Read the model definition and answer for the solid it produces. Units are mm, in the model's axes. Face numbers are marked on the shaded views. A direction names the side the tool comes from. Coordinates: 2 decimals unless noted, no trailing zeros. Write each loop counter-clockwise with the first axis right and the second up, starting at its lowest first coordinate (ties: lowest second). Pieces come first, ordered by that corner, then holes.
Item 1: Section C-C (z = -3.5) is taken. Give the vertices of the cut face in (x, y).
Item 2: Straight lines are drawn through the part: probe 1 along Y at (x, z) = (3.5, 2); probe 2 along X at (y, z) = (-30, 7.75); probe 3 along X at (y, z) = (24, 6). For each, find the intervals that lie inside material, in ascending order.
Item 3: Section D-D (x = -20) is taken. Give the vertices of the cut face in (y, z), then the cut area to 3 significant figures.
Item 4: Section A-A (z = 8.5) is taken. State how many separate pieces and enclosed holes the cut face has, then the cut area to 3 significant figures.
Item 5: Determine the mould class of the marked faces 6, 7, 8 and 9 for opening direction X: released by +X, released by -X, zero draft, split by the parting line, or undercut.
Item 6: A tool of negligible diameter and unlimited length cuts with its end or side. For the marked faces 1, 2, 3, 4 and 5, from which of +Z, -Z, +X, -X, +Y, -Y can it reach the whole face along a straight path? Write none if from no direction.
Item 7: Each of these flat-tipped pins is pushed along its axis until it touches: P1, Ø6, axis at x = -20, y = -30, coming from the +Z side; P2, Ø8, axis at x = 17, z = -2.5, coming from the -Y side; P3, Ø10, axis at x = -2, y = 20, coming from the +Z side; P4, Ø3, axis at x = -2, y = 26, coming from the -Z side. Where does it stop, or does it pass through?
Item 8: Section B-B (y = 8) is taken. Give the vertices of the cut face in (x, z), then the cut area to 3 significant figures.
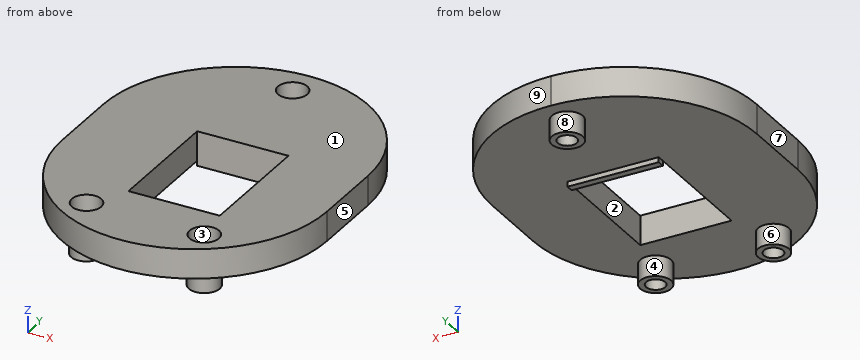
from build123d import *

# Parameters (mm, degrees)
F1_DEPTH    = 10
F3_R        = 44.99999
F4_W        = 31
F4_H        = 42
F5_DEPTH    = 11
F6_R        = 5.25
F7_DEPTH    = 7
F9_D        = 10
F9_DEPTH    = 10.001
F10_D       = 6.5
F10_ON_F6_D = 6.5
F11_W       = 31
F11_H       = 2.5
F12_DEPTH   = 1.7


# Not quite as in the source:
# - a fillet or chamfer is up to 0.001 mm smaller than in the source, because OpenCascade refuses the exact size


with BuildPart() as f1:
    # F0 (on Top) → F1 (new body)
    with BuildSketch(Plane.XY):
        with BuildLine():
            Line((-45, 70), (-45, 0))
            ThreePointArc((-45, 0), (0, -45), (45, 0))
            Line((45, 0), (45, 70))
            Line((45, 70), (-45, 70))
        make_face()
    extrude(amount=F1_DEPTH)

    # F3 (radius 45 in the source; OpenCascade refuses exactly that, so slightly less here)
    f3_edges = [f1.edges().sort_by_distance(p)[0] for p in [
        (-45, 70, 5),
        (45, 70, 5),
    ]]
    fillet(f3_edges, radius=F3_R)

    # F4 (on face) → F5 (cut)
    with BuildSketch(Plane.XY.offset(10)):
        with Locations((2.9, 3.3)):
            Rectangle(F4_W, F4_H)
    extrude(amount=-F5_DEPTH, mode=Mode.SUBTRACT)

    # F6 (on face) → F7 (join)
    with BuildSketch(Plane(origin=(0, 0, 0), x_dir=(1, 0, 0), z_dir=(0, 0, -1))):
        with Locations((0, -60)):
            Circle(F6_R)
        with Locations((-20, 30)):
            Circle(F6_R)
        with Locations((20, 30)):
            Circle(F6_R)
    extrude(amount=F7_DEPTH)

    # F9 (through all, one way)
    with BuildSketch(Plane(origin=(0, 0, 0), x_dir=(1, 0, 0), z_dir=(0, 0, -1))):
        with Locations((-20, 30), (20, 30), (0, -60)):
            Circle(F9_D / 2)
    extrude(amount=-F9_DEPTH, mode=Mode.SUBTRACT)

    # F10 (through all)
    with Locations(Plane.XY):
        with Locations((20, -30), (0, 60)):
            Hole(F10_D / 2)

    # F10 on F6 (through all)
    with Locations(Plane.XY):
        with Locations((-20, -30)):
            Hole(F10_ON_F6_D / 2)

    # F11 (on face) → F12 (join)
    with BuildSketch(Plane(origin=(0, 0, 0), x_dir=(1, 0, 0), z_dir=(0, 0, -1))):
        with Locations((2.9, -25.55)):
            Rectangle(F11_W, F11_H)
    extrude(amount=F12_DEPTH)


solid = f1.part
Established:
1. outline: circle Ø10.5 at (-20, -30); circle Ø10.5 at (0, 60); circle Ø10.5 at (20, -30); hole circle Ø6.5 at (-20, -30); hole circle Ø6.5 at (0, 60); hole circle Ø6.5 at (20, -30)
2. probe 1: y = -44.86 to -17.7, 24.3 to 56.43, 63.57 to 69.86
2. probe 2: x = -33.54 to -25, -15 to 15, 25 to 33.54
2. probe 3: x = -45 to -12.6, 18.4 to 45
3. outline: (-40.31, 0) - (-35.25, 0) - (-35.25, -7) - (-33.25, -7) - (-33.25, 0) - (-35, 0) - (-35, 10) - (-40.31, 10) - close; (-26.75, -7) - (-24.75, -7) - (-24.75, 0) - (65.31, 0) - (65.31, 10) - (-25, 10) - (-25, 0) - (-26.75, 0) - close
3. area: 984 mm2
4. separate pieces: 1
4. enclosed holes: 4
4. area: 7,070 mm2
5. face 6: undercut
5. face 7: released by -X
5. face 8: split by the parting line
5. face 9: released by +X
6. face 1: +Z, +X, -X, +Y, -Y
6. face 2: +Z, -Z
6. face 3: +Z
6. face 4: -Z
6. face 5: +Z, -Z, +X, +Y, -Y
7. P1: passes through
7. P2: stops at y = -42.81
7. P3: stops at z = 10
7. P4: stops at z = -1.7
8. outline: (-45, 0) - (-12.6, 0) - (-12.6, 10) - (-45, 10) - close; (18.4, 0) - (45, 0) - (45, 10) - (18.4, 10) - close
8. area: 590 mm2
